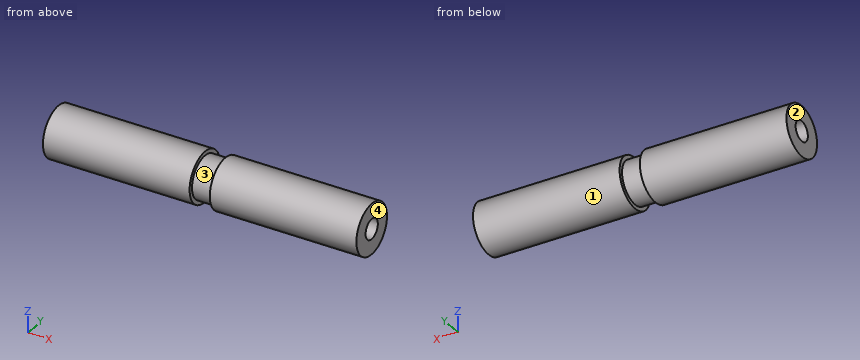
Autodesk Inventor part; units mm, degrees
ref_plane "YZ Plane" through (0, 0, 0) normal (1, 0, 0) x (0, 1, 0)
ref_plane "XZ Plane" through (0, 0, 0) normal (0, 1, 0) x (-1, 0, 0)
ref_plane "XY Plane" through (0, 0, 0) normal (0, 0, 1) x (1, 0, 0)
sketch "Sketch1" plane through (0, 0, 0) normal (1, 0, 0) x (0, 1, 0)
  circle A0 centre (0, 0) radius 3.175
  dimension "d0" = 6.35
extrude "Extrusion1" add sketch "Sketch1" along normal blind 39.37
sketch "Sketch2" plane through (39.37, 0, 0) normal (1, 0, 0) x (0, 0, -1)
  circle A0 centre (0, 0) radius 1.27
  dimension "d3" = 2.54
extrude "Extrusion2" cut sketch "Sketch2" against normal blind 39.37
thread "Thread1"
sketch "Sketch5" plane through (0, 0, 0) normal (0, 1, 0) x (-1, 0, 0)
  line L0 (0, 0) -> (-39.37, 0)
  line L1 (-39.37, 3.175) -> (-39.37, -3.175)
  line L2 (0, -3.175) -> (-39.37, -3.175)
  line L3 (-19.685, -3.175) -> (-18.415, -3.175)
  line L4 (-18.415, -3.175) -> (-18.415, -2.667)
  line L5 (-18.415, -2.667) -> (-20.955, -2.667)
  line L6 (-20.955, -2.667) -> (-20.955, -3.175)
  line L7 (-20.955, -3.175) -> (-19.685, -3.175)
  dimension "d11" = 1.27
  dimension "d12" = 0.508
  dimension "d13" = 2.54
revolve "Revolution1" cut sketch "Sketch5" angle 360 about axis through (0, 0, 0) along (1, 0, 0)
properties part number "clawholder"
Geometry check sheet. Reference: the model listing, model coordinates, mm. Face numbers are marked on the shaded views. Coordinates: 2 decimals unless noted, no trailing zeros. Write each loop counter-clockwise with the first axis right and the second up, starting at its lowest first coordinate (ties: lowest second). Pieces come first, ordered by that corner, then holes. Notation, with made-up numbers: M 20,7 L 70,7 A34 ccw 70,44 Z; hole C 79,-3 d2. An arc over 180 degrees is marked long. One line per item, written item: value. Start each with the question number.
(1) Scan lines: line 1 along Y through (x, z) = (20, 0); line 2 along X through (y, z) = (1.75, -2.25) (3 decimals); line 3 along Y through (x, z) = (15, 0) (3 decimals). Record each from-to range of solid material in increasing order. Write a range as [from, to].
(2) Sectioned sample at D-D, the plane z = 1.75. Enter the section's corners in (x, y) (3 decimals), and give its area (3 significant figures).
(3) Depth check by flat-ended pin: pin 1 (3 mm diameter, centred on x = 27, z = 2, fed in from +Y). Enter the tip coordinate at first touch or a pass-through.
(4) Release check for a two-part mould opening along X. For the marked faces 1, 2, 3 and 4 record: released by +X, released by -X, zero draft, split by the parting line, or undercut.
(5) Sectioned sample at A-A, the plane y = 0. Enter the section's corners in (x, z) (3 decimals), and give its area (3 significant figures).
(6) Sectioned sample at C-C, the plane x = 10.5. Enter the section's corners in (y, z) (3 decimals), and give its area (3 significant figures).
Filled sheet:
1. line 1: [-2.67, -1.27], [1.27, 2.67]
1. line 2: [0, 18.415], [20.955, 39.37]
1. line 3: [-3.175, -1.27], [1.27, 3.175]
2. outline: M 0,-2.649 L 18.415,-2.649 L 18.415,-2.013 L 20.955,-2.013 L 20.955,-2.649 L 39.37,-2.649 L 39.37,2.649 L 20.955,2.649 L 20.955,2.013 L 18.415,2.013 L 18.415,2.649 L 0,2.649 Z
2. area: 205 mm²
3. pin 1: y = 3.14
4. face 1: zero draft
4. face 2: released by -X
4. face 3: undercut
4. face 4: released by +X
5. outline: M 0,-3.175 L 18.415,-3.175 L 18.415,-2.667 L 20.955,-2.667 L 20.955,-3.175 L 39.37,-3.175 L 39.37,-1.27 L 0,-1.27 Z; M 0,1.27 L 39.37,1.27 L 39.37,3.175 L 20.955,3.175 L 20.955,2.667 L 18.415,2.667 L 18.415,3.175 L 0,3.175 Z
5. area: 147 mm²
6. outline: C 0,0 d6.35; hole C 0,0 d2.54
6. area: 26.6 mm²
